Input: part model. Units: mm. Frame: model coordinates. A direction names the side the tool comes from. Give positions to 0.01 mm unless a question says otherwise; leave off trailing zeros. Loops run counter-clockwise (first coordinate to the right, second up) from the corner with the lowest first, then second, coordinate; pieces in that order, holes last. Notation, with made-up numbers: (-11, 3.5) -> (38, 3.5) arc R16 ccw to (38, 31.5) -> close; hole circle Ø8 at (28.25, 81.25). An arc over 180 degrees is marked (long way). Answer as a JSON object with one key per item and string values. Group by question number.
```python
from build123d import *

# Parameters (mm, degrees)
SKETCH1_W           = 50
SKETCH1_H           = 25
BOSS_EXTRUDE1_DEPTH = 5
SKETCH2_W           = 14.5
SKETCH2_H           = 16
CUT_EXTRUDE1_DEPTH  = 5
SKETCH3_W           = 14.6
SKETCH3_H           = 16.1
CUT_EXTRUDE2_DEPTH  = 5
SKETCH5_W           = 3
SKETCH5_H           = 1
SKETCH5_W_2         = 6
CUT_EXTRUDE3_DEPTH  = 1
SKETCH6_W           = 50
SKETCH6_H           = 25
BOSS_EXTRUDE2_DEPTH = 5
SKETCH7_W           = 16.25
SKETCH7_H           = 14.5
CUT_EXTRUDE4_DEPTH  = 4
SKETCH8_W           = 14.75
SKETCH8_H           = 14.5
CUT_EXTRUDE5_DEPTH  = 1
SKETCH9_W           = 2.5
SKETCH9_H           = 14
BOSS_EXTRUDE3_DEPTH = 4.6
SKETCH10_W          = 5
SKETCH10_H          = 14
BOSS_EXTRUDE4_DEPTH = 2.5
BOSS_EXTRUDE5_DEPTH = 14
FILLET1_R           = 1
SKETCH12_W          = 2
SKETCH12_H          = 14
BOSS_EXTRUDE6_DEPTH = 6
FILLET2_R           = 4
FILLET3_R           = 1
FILLET4_R           = 0.5
SKETCH13_W          = 14
SKETCH13_H          = 2.5
CUT_EXTRUDE6_DEPTH  = 0.5


with BuildPart() as part:
    # Sketch1 → Boss-Extrude1 (new body)
    with BuildSketch(Plane(origin=(0, 0, 0), x_dir=(1, 0, 0), z_dir=(0, 1, 0))):
        Rectangle(SKETCH1_W, SKETCH1_H)
    extrude(amount=BOSS_EXTRUDE1_DEPTH)

    # Sketch2 → Cut-Extrude1 (cut)
    with BuildSketch(Plane(origin=(0, 5, 0), x_dir=(1, 0, 0), z_dir=(0, 1, 0))):
        with Locations((-12.821632497, -0.096290121)):
            Rectangle(SKETCH2_W, SKETCH2_H)
    extrude(amount=-CUT_EXTRUDE1_DEPTH, mode=Mode.SUBTRACT)

    # Sketch3 → Cut-Extrude2 (cut)
    with BuildSketch(Plane(origin=(0, 5, 0), x_dir=(1, 0, 0), z_dir=(0, 1, 0))):
        with Locations((11.118853314, -0.27633095)):
            Rectangle(SKETCH3_W, SKETCH3_H)
    extrude(amount=-CUT_EXTRUDE2_DEPTH, mode=Mode.SUBTRACT)

    # Sketch5 → Cut-Extrude3 (cut)
    with BuildSketch(Plane(origin=(0, 5, 0), x_dir=(1, 0, 0), z_dir=(0, 1, 0))):
        with Locations((-12.529830787, 10.403858803)):
            Rectangle(SKETCH5_W, SKETCH5_H)
        with Locations((12.528710417, 10.30293358)):
            Rectangle(SKETCH5_W_2, SKETCH5_H)
    extrude(amount=-CUT_EXTRUDE3_DEPTH, mode=Mode.SUBTRACT)

    # Sketch6 → Boss-Extrude2 (add)
    with BuildSketch(Plane(origin=(0, 0, 0), x_dir=(1, 0, 0), z_dir=(0, 1, 0))):
        with Locations((0, -25)):
            Rectangle(SKETCH6_W, SKETCH6_H)
    extrude(amount=BOSS_EXTRUDE2_DEPTH)

    # Sketch7 → Cut-Extrude4 (cut)
    with BuildSketch(Plane(origin=(0, 5, 0), x_dir=(1, 0, 0), z_dir=(0, 1, 0))):
        with Locations((-1.214601825, -24.398968546)):
            Rectangle(SKETCH7_W, SKETCH7_H)
    extrude(amount=-CUT_EXTRUDE4_DEPTH, mode=Mode.SUBTRACT)

    # Sketch8 → Cut-Extrude5 (cut)
    with BuildSketch(Plane(origin=(0, 1, 0), x_dir=(1, 0, 0), z_dir=(0, 1, 0))):
        with Locations((-1.964601825, -24.398968546)):
            Rectangle(SKETCH8_W, SKETCH8_H)
    extrude(amount=-CUT_EXTRUDE5_DEPTH, mode=Mode.SUBTRACT)

    # Sketch9 → Boss-Extrude3 (add)
    with BuildSketch(Plane(origin=(0, 5, 0), x_dir=(1, 0, 0), z_dir=(0, 1, 0))):
        with Locations((13.660398175, -24.242407708)):
            Rectangle(SKETCH9_W, SKETCH9_H)
    extrude(amount=BOSS_EXTRUDE3_DEPTH)

    # Sketch10 → Boss-Extrude4 (add)
    with BuildSketch(Plane(origin=(0, 9.6, 0), x_dir=(1, 0, 0), z_dir=(0, 1, 0))):
        with Locations((12.410398175, -24.242407708)):
            Rectangle(SKETCH10_W, SKETCH10_H)
    extrude(amount=BOSS_EXTRUDE4_DEPTH)

    # Sketch11 → Boss-Extrude5 (add)
    with BuildSketch(Plane.XY.offset(31.242407708)):
        Polygon((14.910398175, 5), (18.418853314, 5), (14.910398175, 12.1), align=None)
    extrude(amount=-BOSS_EXTRUDE5_DEPTH)

    # Fillet1
    fillet1_edges = [part.edges().sort_by_distance(p)[0] for p in [
        (14.910398175, 12.1, 24.242407708),
        (18.418853314, 5, 24.242407708),
    ]]
    fillet(fillet1_edges, radius=FILLET1_R)

    # Sketch12 → Boss-Extrude6 (add)
    with BuildSketch(Plane(origin=(0, 5, 0), x_dir=(1, 0, 0), z_dir=(0, 1, 0))):
        with Locations((-11.939601825, -24.648968546)):
            Rectangle(SKETCH12_W, SKETCH12_H)
    extrude(amount=BOSS_EXTRUDE6_DEPTH)

    # Fillet2
    fillet2_edges = [part.edges().sort_by_distance(p)[0] for p in [
        (-12.939601825, 5, 24.648968546),
    ]]
    fillet(fillet2_edges, radius=FILLET2_R)

    # Fillet3
    fillet3_edges = [part.edges().sort_by_distance(p)[0] for p in [
        (12.410398175, 5, 24.242407708),
    ]]
    fillet(fillet3_edges, radius=FILLET3_R)

    # Fillet4
    fillet4_edges = [part.edges().sort_by_distance(p)[0] for p in [
        (-10.939601825, 5, 24.648968546),
    ]]
    fillet(fillet4_edges, radius=FILLET4_R)

    # Sketch13 → Cut-Extrude6 (cut)
    with BuildSketch(Plane.ZY.offset(-9.910398175)):
        with Locations((24.242407708, 10.85)):
            Rectangle(SKETCH13_W, SKETCH13_H)
    extrude(amount=-CUT_EXTRUDE6_DEPTH, mode=Mode.SUBTRACT)


solid = part.part
```
Q1. Ray query, probe 1 along X at (y, z) = (4.75, 28); probe 2 along Z at (x, y) = (-19.5, 3.25); probe 3 along Z at (x, y) = (11.5, 4.75). Return the intervals inside material, ascending.
Q2. Section A-A on z = 21. Return the cut outline in (x, y), then the cut area to 3 significant figures.
Q3. Section B-B on y = 3. Return the cut outline in (x, z), then the cut area to 3 significant figures.
Q4. Section D-D on x = 0. Return the cut outline in (y, z), then the cut area to 4 significant figures.
Q5. Pin query (flat end, axial travel): pin 1 Ø1 at (y, z) = (6.5, 26.5) entering from +X; pin 2 Ø2 at (x, y) = (16.5, 8.5) entering from +Z; pin 3 Ø1.1 at (x, z) = (14, -10) entering from +Y. Return the tip coordinate at first contact, or that it passes through.
Q6. Section C-C on z = -4. Return the cut outline in (x, y), then the cut area to 4 significant figures.
Q7. Set-up query: faces 4 (the face through (-9.34, 3, 25)), 5 (the face through (12.41, 8, 24)), 6 (the face through (10.41, 11, 24)), 7 (the face through (-12, 11, 25)), 8 (the face through (14, 9, 31.242)). Return all of +Z, -Z, +X, -X, +Y, -Y with unobstructed straight access to the full face (end or side cutting, diameter ignored); none if empty.
Q8. Pull-direction query (Y, two-part tool) for faces 1 (the face through (11, 9.6, 24)), 2 (the face through (-1, 3, 31.649)), 3 (the face through (-14.142, 6.141, 24.551)); classes: +Y half, -Y half, draft (parallel to the pull), parting line (faces both ways), or undercut.
Numbers:
{
 "1": {"probe 1": "x = -25 to -9.34, 6.91 to 25", "probe 2": "z = -12.5 to -7.9, 8.1 to 37.5", "probe 3": "z = -12.5 to -10.8, -9.8 to -7.77, 8.33 to 37.5"},
 "2": {"outline": "(-25, 0) -> (-9.34, 0) -> (-9.34, 5) -> (-10.44, 5) arc R0.5 cw to (-10.94, 5.5) -> (-10.94, 11) -> (-12.94, 11) -> (-12.94, 9) arc R4 cw to (-16.94, 5) -> (-25, 5) -> close; (5.41, 0) -> (25, 0) -> (25, 5) -> (19.04, 5) arc R1 cw to (18.14, 5.56) -> (15.19, 11.54) arc R1 ccw to (14.29, 12.1) -> (10.41, 12.1) -> (10.41, 9.6) -> (12.41, 9.6) -> (12.41, 6) arc R1 cw to (11.41, 5) -> (6.91, 5) -> (6.91, 1) -> (5.41, 1) -> close", "area": "221 mm²"},
 "3": {"outline": "(-25, -12.5) -> (25, -12.5) -> (25, 37.5) -> (-25, 37.5) -> close; hole (-20.07, -7.9) -> (-5.57, -7.9) -> (-5.57, 8.1) -> (-20.07, 8.1) -> close; hole (-9.34, 17.15) -> (6.91, 17.15) -> (6.91, 31.65) -> (-9.34, 31.65) -> close; hole (3.82, -7.77) -> (18.42, -7.77) -> (18.42, 8.33) -> (3.82, 8.33) -> close", "area": "1,800 mm²"},
 "4": {"outline": "(0, -12.5) -> (5, -12.5) -> (5, 17.15) -> (0, 17.15) -> close; (0, 31.65) -> (5, 31.65) -> (5, 37.5) -> (0, 37.5) -> close", "area": "177.5 mm²"},
 "5": {"pin 1": "stops at x = 17.92", "pin 2": "stops at z = 31.24", "pin 3": "stops at y = 5"},
 "6": {"outline": "(-25, 0) -> (-20.07, 0) -> (-20.07, 5) -> (-25, 5) -> close; (-5.57, 0) -> (3.82, 0) -> (3.82, 5) -> (-5.57, 5) -> close; (18.42, 0) -> (25, 0) -> (25, 5) -> (18.42, 5) -> close", "area": "104.5 mm²"},
 "7": {"face 4": "+Y, -Y", "face 5": "+Z, -Z", "face 6": "+Z, -Z, +Y", "face 7": "+Z, -Z, -X, +Y", "face 8": "+Z, +X, +Y"},
 "8": {"face 1": "undercut", "face 2": "draft", "face 3": "+Y half"}
}
